Autodesk Inventor part; units mm, degrees
ref_plane "Cross Section Plane" through (311.7698, 156.3537, 0) normal (-0.9855, -0.1698, 0) x (0, 0, 1)
ref_plane "YZ Plane" through (0, 0, 0) normal (1, 0, 0) x (0, 1, 0)
ref_plane "XZ Plane" through (0, 0, 0) normal (0, 1, 0) x (-1, 0, 0)
sketch "Sketch Path" plane through (0, 0, 0) normal (0, 0, 1) x (1, 0, 0)
  arc A0 (325.3537, 77.5154) -> (311.7698, 156.3537) centre (318.5618, 116.9345) ccw
  arc A1 (-225.3064, 63.8154) -> (-211.7226, -15.0229) centre (-218.5145, 24.3963) ccw
  line L0 (-225.3064, 63.8154) -> (311.7698, 156.3537)
  line L1 (325.3537, 77.5154) -> (-211.7226, -15.0229)
ref_plane "Cross Section Plane" through (311.7698, 156.3537, 0) normal (-0.9855, -0.1698, 0) x (0, 0, 1)
sketch "Cross Section" plane through (311.7698, 156.3537, 0) normal (-0.9855, -0.1698, 0) x (0, 0, 1)
  line L0 (0, 2.4986) -> (0, -3.5014) construction
  line L1 (-4.25, 0) -> (4.25, 0) construction
  line L2 (-5.1594, 2.4986) -> (5.1594, 2.4986)
  line L3 (5.1594, 2.4986) -> (2.9756, -3.5014)
  line L4 (2.9756, -3.5014) -> (-2.9756, -3.5014)
  line L5 (-2.9756, -3.5014) -> (-5.1594, 2.4986)
  point P0 (0, 0)
  point P1 (0, 0)
  point P2 (0, 0)
  dimension "d0" = 8.5
  dimension "d1" = 2.4986
  dimension "d2" = 40
  dimension "d3" = 6
sweep "Belt" add profiles "Cross Section" path "Sketch Path"
equation "\"d0\" = da_Bw"
equation "\"d1\" = da_Hw"
equation "\"d2\" = da_Alfa"
equation "\"d3\" = da_H"
equation "\"da_Alfa\" = 40deg"
equation "\"da_H\" = 6"
equation "\"da_Bw\" = 8.5"
equation "\"da_Hw\" = 2.49859"
properties part number "V-Belt" material "Rubber"
Read the model definition and answer for the solid it produces. Units are mm, in the model's axes. A direction names the side the tool comes from. Round coordinates to 2 decimals unless told otherwise and drop trailing zeros. Write each loop counter-clockwise with the first axis right and the second up, starting at its lowest first coordinate (ties: lowest second). Pieces come first, ordered by that corner, then holes.
1. Which of the six approach directions +Z, -Z, +X, -X, +Y, -Y give full straight-line access (tool end or side, diameter ignored) to faces 5 (the face through (60.5, 32.3, -4.1)), 6 (the face through (39.05, 111.9, 0.07)), 7 (the face through (-254.98, 18.94, 3.11)), 8 (the face through (40.067, 105.986, -0.042))?
2. Determine the mould class of faces 1 (the face through (61, 29.43, 0.07)), 2 (the face through (39.56, 108.9, 4.05)), 3 (the face through (354.75, 123.99, -3.11)), 4 (the face through (-260.227, 16.261, -0.072)) for opening direction Y: pulls with the +Y half, pulls with the -Y half, needs draft (parallel to the pull), parting line crosses it, or undercut.
3. Straight lines are drawn through the part: L1, parallel to Y at x = -199.5, z = -0.5; L2, parallel to Y at x = 18.5, z = 1; L3, parallel to Z at x = 209, y = 60.5. For each, find the intervals that lie inside material, in ascending order.
4. Given pin 1 Ø4 at (x, z) = (293.5, 1) entering from +Y; pin 2 Ø2 at (x, z) = (190, -1) entering from +Y; pin 3 Ø1 at (y, z) = (104, -3) entering from +X, each flat-ended and moving along its own axis, determine where each tip first touches the part or whether it passes through.
5. The part is cut by section B-B, the plane x = -125.5. Determine the outline of the cut face in (y, z), then the cut area to 3 significant figures.
Values:
1. face 5: -Z
1. face 6: +Z, -Z, -X, +Y
1. face 7: +Z
1. face 8: +Z, -Z
2. face 1: pulls with the -Y half
2. face 2: undercut
2. face 3: undercut
2. face 4: parting line crosses it
3. L1: y = -15.45 to -9.36, 64.71 to 70.8
3. L2: y = 22.11 to 28.2, 102.27 to 108.36
3. L3: z = -3.16 to 3.16
4. pin 1: stops at y = 156.09
4. pin 2: stops at y = 138.08
4. pin 3: stops at x = 359.2
5. outline: (-2.7, -5.16) - (3.39, -2.98) - (3.39, 2.98) - (-2.7, 5.16) - close; (77.46, -2.98) - (83.55, -5.16) - (83.55, 5.16) - (77.46, 2.98) - close
5. area: 99.1 mm2
